Autodesk Inventor part; units mm, degrees
ref_plane "YZ Plane" through (0, 0, 0) normal (1, 0, 0) x (0, 1, 0)
ref_plane "XZ Plane" through (0, 0, 0) normal (0, 1, 0) x (-1, 0, 0)
ref_plane "XY Plane" through (0, 0, 0) normal (0, 0, 1) x (1, 0, 0)
sketch "Sketch1" plane through (0, 0, 0) normal (0, 0, 1) x (1, 0, 0)
  arc A0 (4.15, 0) -> (-4.15, 0) centre (0, 0) ccw
  line L0 (-21.6509, 0) -> (19.2313, 0)
  line L1 (-13, 0) -> (-13, 5.15)
  line L2 (-13, 5.15) -> (13, 5.15)
  line L3 (13, 5.15) -> (13, 0)
  line L4 (-13, 0) -> (-4.15, 0)
  line L5 (4.15, 0) -> (13, 0)
  dimension "d0" = 8.3
  dimension "d1" = 1
  dimension "d2" = 13
  dimension "d3" = 13
extrude "Extrusion1" add sketch "Sketch1" along normal blind 20 contours A0 L0 L1 L2 L3
sketch "Sketch2" plane through (-13, 5.15, 0) normal (0, 1, 0) x (1, 0, 0)
  line L0 (-4.8106, -10) -> (24.391, -10) construction
  line L1 (26, 0) -> (0, 0) construction
  line L2 (26, -20) -> (0, -20) construction
  circle A0 centre (5, -10) radius 1.9
  circle A1 centre (21, -10) radius 1.9
  point P0 (13, 0)
  dimension "d7" = 20
  dimension "d8" = 10
  dimension "d9" = 3.8
  dimension "d10" = 3.8
  dimension "d11" = 16
  dimension "d12" = 8
extrude "Extrusion2" cut sketch "Sketch2" against normal through all
sketch "Sketch3" plane through (-13, 0, 0) normal (0, -1, 0) x (1, 0, 0)
  line L0 (0, 0) -> (0, 20)
  line L1 (0, 2) -> (2, 2)
  line L2 (2, 2) -> (2, 18)
  line L3 (2, 18) -> (0, 18)
  line L4 (0, 18) -> (0, 2)
  line L5 (26, 0) -> (26, 20)
  line L6 (26, 2) -> (24, 2)
  line L7 (24, 2) -> (24, 18)
  line L8 (24, 18) -> (26, 18)
  line L9 (26, 18) -> (26, 2)
  line L10 (0, 0) -> (8.85, 0)
  line L11 (0, 20) -> (8.85, 20)
  line L12 (17.15, 20) -> (26, 20)
  line L13 (17.15, 0) -> (26, 0)
  point P0 (13, 0)
  point P1 (0, 18)
  dimension "d15" = 2
  dimension "d16" = 2
  dimension "d17" = 2
  dimension "d18" = 2
  dimension "d19" = 2
  dimension "d20" = 2
extrude "Extrusion3" cut sketch "Sketch3" against normal blind 2
chamfer "Chamfer1" distance 0.5 angle 45 4 edges at (13, 5.15, 10) (0, 5.15, 20) (-13, 5.15, 10) (0, 5.15, 0)
equation "\"d8\" = 0.5 * d7"
equation "\"d10\" = d9"
equation "\"d16\" = d15"
equation "\"d17\" = d15"
equation "\"d18\" = d16"
equation "\"d19\" = d16"
equation "\"d20\" = d17"
properties part number "_3DPrint"
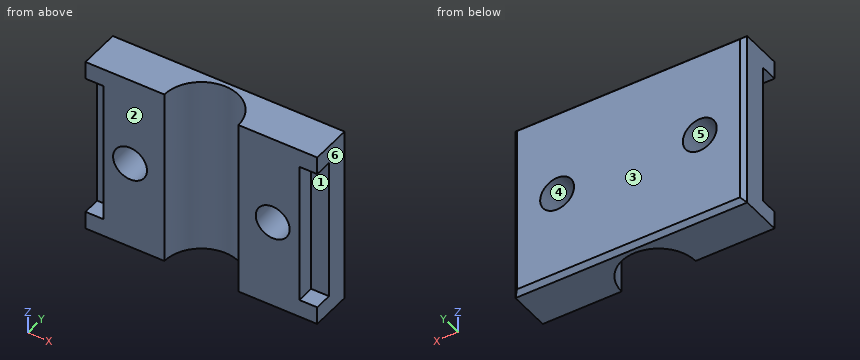
Here's how the part is built. I have some questions about the finished solid (model axes, mm). Face numbers are marked on the shaded views. A direction names the side the tool comes from. Coordinates: 2 decimals unless noted, no trailing zeros. Write each loop counter-clockwise with the first axis right and the second up, starting at its lowest first coordinate (ties: lowest second). Pieces come first, ordered by that corner, then holes. Notation, with made-up numbers: (37.25, 22) -> (50.25, 22) arc R35 ccw to (50.25, 60) -> close; hole circle Ø9 at (34.5, 20.25). An arc over 180 degrees is marked (long way). Use a Markdown table: item, result. Add a question column.
(1) Please list where these lines run through material, in increasing order: line 1 (Z direction, x = 8, y = 3); line 2 (X direction, y = 3.25, z = 10); line 3 (X direction, y = 2.3, z = 10).
(2) For the marked faces 1 and 2, which set-ups out of +Z, -Z, +X, -X, +Y, -Y let a thin tool reach every point of the face, with its end or its side?
(3) If we section it at C-C, the plane x = 8: Write out the boundary of the cut face in (y, z).
(4) I'm going to push flat-ended pins straight in: P1, Ø3, axis at x = 8, z = 10, coming from the +Y side; P2, Ø1.6, axis at y = 1, z = 8, coming from the +X side; P3, Ø1.6, axis at y = 0.5, z = 13.5, coming from the -X side; P4, Ø1.6, axis at x = -12, z = 12.5, coming from the -Y side. Where does each tip first touch, or does it pass through?
(5) If we section it at B-B, the plane z = 10: Write out the boundary of the cut face in (x, y), and give its area (3 significant figures).
(6) We'd pull the mould along X, two halves only. Please class the marked faces 3, 4, 5 and 6: +X half, -X half, draft (parallel to the pull), parting line (faces both ways), or undercut.
(7) If we section it at A-A, the plane y = 2.3: Write out the boundary of the cut face in (x, z).
(8) If we section it at D-D, the plane y = 0.4: Write out the boundary of the cut face in (x, z).
Outcome:
| question | item | result |
|---|---|---|
| 1 | line 1 | z = 0 to 8.1, 11.9 to 20 |
| 1 | line 2 | x = -13 to -9.9, -6.1 to -2.58, 2.58 to 6.1, 9.9 to 13 |
| 1 | line 3 | x = -13 to -9.9, -6.1 to -3.45, 3.45 to 6.1, 9.9 to 13 |
| 2 | face 1 | +X, -Y |
| 2 | face 2 | +Z, -Z, +X, -X, -Y |
| 3 | outline | (0, 0) -> (4.65, 0) -> (5.15, 0.5) -> (5.15, 8.1) -> (0, 8.1) -> close; (0, 11.9) -> (5.15, 11.9) -> (5.15, 19.5) -> (4.65, 20) -> (0, 20) -> close |
| 4 | P1 | passes through |
| 4 | P2 | stops at x = 11 |
| 4 | P3 | stops at x = -11 |
| 4 | P4 | stops at y = 2 |
| 5 | outline | (-13, 2) -> (-11, 2) -> (-11, 0) -> (-9.9, 0) -> (-9.9, 5.15) -> (-12.5, 5.15) -> (-13, 4.65) -> close; (-6.1, 0) -> (-4.15, 0) arc R4.15 cw to (4.15, 0) -> (6.1, 0) -> (6.1, 5.15) -> (-6.1, 5.15) -> close; (9.9, 0) -> (11, 0) -> (11, 2) -> (13, 2) -> (13, 4.65) -> (12.5, 5.15) -> (9.9, 5.15) -> close |
| 5 | area | 59.5 mm^2 |
| 6 | face 3 | draft |
| 6 | face 4 | undercut |
| 6 | face 5 | undercut |
| 6 | face 6 | +X half |
| 7 | outline | (-13, 0) -> (-3.45, 0) -> (-3.45, 20) -> (-13, 20) -> close; (3.45, 0) -> (13, 0) -> (13, 20) -> (3.45, 20) -> close; hole circle Ø3.8 at (-8, 10); hole circle Ø3.8 at (8, 10) |
| 8 | outline | (-13, 0) -> (-4.13, 0) -> (-4.13, 20) -> (-13, 20) -> (-13, 18) -> (-11, 18) -> (-11, 2) -> (-13, 2) -> close; (4.13, 0) -> (13, 0) -> (13, 2) -> (11, 2) -> (11, 18) -> (13, 18) -> (13, 20) -> (4.13, 20) -> close; hole circle Ø3.8 at (-8, 10); hole circle Ø3.8 at (8, 10) |
